Design review of the part built by this model. Coordinates are the model's own, in mm. A direction names the side the tool comes from. Coordinates: 2 decimals unless noted, no trailing zeros. Use a Markdown table: item, result. Add a question column.
Q1. Draft analysis for pull direction X (two halves, no side actions). For faces 1 (the face through (3, 14, -1)), 2 (the face through (3.393, 6.902, 1.111)), 3 (the face through (0.01, 6.9, -3.57)), state which applies: pulls with the +X half, pulls with the -X half, needs draft (parallel to the pull), parting line crosses it, or undercut.
Q2. For faces 4 (the face through (-3.03, 6.902, -2.707)), 5 (the face through (3.398, 6.902, -1.095)), 6 (the face through (-2, 14.5, 1)), 7 (the face through (-1.64, 6.9, -3.73)), list the 3-axis set-ups (+Z, -Z, +X, -X, +Y, -Y) from which the entire face can be reached by the end or side of a thin tool; tool diameter is ignored.
Q3. For probe 1 along Z at (x, y) = (0, 9.75); probe 2 along Z at (x, y) = (3.75, 12); probe 3 along Z at (x, y) = (3.25, 12.75), list the stretches that pass through material, from the lowest coordinate up.
Q4. Clearance check with flat-ended pins moving along their axes: pin 1 Ø4 at (x, y) = (1.5, 9) entering from +Z; pin 2 Ø2 at (x, z) = (0, -3.5) entering from +Y; pin 3 Ø3 at (y, z) = (3, 3) entering from +X. State where each tip first meets the part, or that it passes through.
from build123d import *

# Parameters (mm, degrees)
BOSS_EXTRUDE3_DEPTH = 14
CIRPATTERN2_COUNT   = 10
SKETCH3_R           = 2.75
BOSS_EXTRUDE4_DEPTH = 0.5
SKETCH4_R           = 2.75
BOSS_EXTRUDE5_DEPTH = 0.5
SKETCH5_R           = 2
BOSS_EXTRUDE6_DEPTH = 2
SKETCH6_R           = 2
BOSS_EXTRUDE7_DEPTH = 2
CHAMFER1_SIZE       = 0.2
SKETCH7_R           = 0.6
CUT_EXTRUDE1_DEPTH  = 20


with BuildPart() as part:
    # Sketch1 → Boss-Extrude3 (new body)
    with BuildSketch(Plane(origin=(0, 0, 0), x_dir=(1, 0, 0), z_dir=(0, 1, 0))):
        with BuildLine():
            ThreePointArc((3.529675716, 0.535060126), (-3.57, 0), (3.529675716, -0.535060126))
            Line((3.529675716, -0.535060126), (3.265358075, -0.599863853))
            ThreePointArc((3.265358075, -0.599863853), (3.32, 0), (3.265358075, 0.599863853))
            Line((3.265358075, 0.599863853), (3.529675716, 0.535060126))
        make_face()
        with BuildLine():
            Line((3.265358075, -0.599863853), (3.529675716, -0.535060126))
            ThreePointArc((3.529675716, -0.535060126), (3.559904655, -0.268288737), (3.57, 0))
            ThreePointArc((3.57, 0), (3.559904655, 0.268288737), (3.529675716, 0.535060126))
            Line((3.529675716, 0.535060126), (3.265358075, 0.599863853))
            ThreePointArc((3.265358075, 0.599863853), (3.32, 0), (3.265358075, -0.599863853))
        make_face()
        with BuildLine():
            Line((4.57, -0.28), (4.57, 0))
            Line((4.57, 0), (4.57, 0.28))
            Line((4.57, 0.28), (3.529675716, 0.535060126))
            ThreePointArc((3.529675716, 0.535060126), (3.559904655, 0.268288737), (3.57, 0))
            ThreePointArc((3.57, 0), (3.559904655, -0.268288737), (3.529675716, -0.535060126))
            Line((3.529675716, -0.535060126), (4.57, -0.28))
        make_face()
    boss_extrude3 = extrude(amount=BOSS_EXTRUDE3_DEPTH)

    # CirPattern2: Boss-Extrude3 ×10 about axis
    cirpattern2_axis = Axis((0, 0, 0), (0, 1, 0))
    for i in range(1, CIRPATTERN2_COUNT):
        add(boss_extrude3.rotate(cirpattern2_axis, i * 360 / CIRPATTERN2_COUNT))

    # Sketch3 → Boss-Extrude4 (add)
    with BuildSketch(Plane(origin=(0, 14, 0), x_dir=(1, 0, 0), z_dir=(0, 1, 0))):
        Circle(SKETCH3_R)
    extrude(amount=BOSS_EXTRUDE4_DEPTH)

    # Sketch4 → Boss-Extrude5 (add)
    with BuildSketch(Plane.XZ):
        Circle(SKETCH4_R)
    extrude(amount=BOSS_EXTRUDE5_DEPTH)

    # Sketch5 → Boss-Extrude6 (add)
    with BuildSketch(Plane(origin=(0, 14.5, 0), x_dir=(1, 0, 0), z_dir=(0, 1, 0))):
        Circle(SKETCH5_R)
    extrude(amount=BOSS_EXTRUDE6_DEPTH)

    # Sketch6 → Boss-Extrude7 (add)
    with BuildSketch(Plane.XZ.offset(0.5)):
        Circle(SKETCH6_R)
    extrude(amount=BOSS_EXTRUDE7_DEPTH)

    # Chamfer1
    chamfer1_edges = [part.edges().sort_by_distance(p)[0] for p in [
        (-2.75, 14.5, 0),
        (-2.75, -0.5, 0),
        (-2, 16.5, 0),
        (-2, -2.5, 0),
    ]]
    chamfer(chamfer1_edges, length=CHAMFER1_SIZE)

    # Sketch7 → Cut-Extrude1 (cut, through all)
    with BuildSketch(Plane.XZ.offset(2.5)):
        Circle(SKETCH7_R)
    extrude(amount=-CUT_EXTRUDE1_DEPTH, mode=Mode.SUBTRACT)


solid = part.part
Answer list:
| question | item | result |
|---|---|---|
| 1 | face 1 | needs draft |
| 1 | face 2 | pulls with the +X half |
| 1 | face 3 | undercut |
| 2 | face 4 | -Z, +Y, -Y |
| 2 | face 5 | +X, +Y, -Y |
| 2 | face 6 | +Y |
| 2 | face 7 | -X, +Y, -Y |
| 3 | probe 1 | -3.57 to -0.6, 0.6 to 3.57 |
| 3 | probe 2 | -2.61 to -2.33, -0.48 to 0.48, 2.33 to 2.61 |
| 3 | probe 3 | -2.8 to -1.74, -1.48 to 1.48, 1.74 to 2.8 |
| 4 | pin 1 | z = 4.43 |
| 4 | pin 2 | y = 14.5 |
| 4 | pin 3 | x = 3.86 |
